from build123d import *

# Parameters (mm, degrees)
F2_R     = 8
F3_SIZE2 = 13
F3_SIZE  = 4


with BuildPart() as f1:
    # F0 (on Top) → F1 (revolve)
    with BuildSketch(Plane.XY):
        with BuildLine():
            Line((-14.3607687205, 22), (-14.3607687205, -20))
            Line((-14.3607687205, -20), (32.0355594158, -20))
            Line((32.0355594158, -20), (32.0355594158, 9.6684019268))
            Line((32.0355594158, 9.6684019268), (52.5324852616, 9.6684019268))
            Line((52.5324852616, 9.6684019268), (52.5324852616, 46.7559769824))
            ThreePointArc((52.5324852616, 46.7559769824), (51.0680191675, 50.2915108883), (47.5324852616, 51.7559769824))
            Line((47.5324852616, 51.7559769824), (16.6392312795, 51.7559769824))
            Line((16.6392312795, 51.7559769824), (16.6392312795, 22))
            Line((16.6392312795, 22), (-14.3607687205, 22))
        make_face()
    revolve(axis=Axis((-14.3607687205, 1, 0), (0, -1, 0)))

    # F2
    f2_edges = [f1.edges().sort_by_distance(p)[0] for p in [
        (-45.360769, 51.755977, 0),
    ]]
    fillet(f2_edges, radius=F2_R)

    # F3
    f3_edges = [f1.edges().sort_by_distance(p)[0] for p in [
        (-60.757097, -20, 0),
    ]]
    chamfer(f3_edges, length=F3_SIZE, length2=F3_SIZE2)


solid = f1.part
For this review, take the finished solid that the model builds, in its own axes (mm). A direction names the side the tool comes from. Round coordinates to 2 decimals unless told otherwise and drop trailing zeros. Order: outer loops, then holes, each group sorted by start corner. A loop starts at its lowest first (then second) coordinate and runs counter-clockwise, first axis right, second up. Notation, with made-up numbers: M -28,40 L -7,40 A26 ccw -7,57 Z; hole C 7.25,56 d5. An arc over 180 degrees is marked long. Use a Markdown table: item, result. Add a question column.
Item 1: Add section A-A, the plane z = 0. Give the boundary of the cut face in (x, y), then the cut area to 3 significant figures.
Item 2: Tool access review of faces 1 (the flat face through (-15, 51.756, -40)), 2 (the cylindrical face through (-60.712, -2.986, 2.04)): name each direction out of +Z, -Z, +X, -X, +Y, -Y from which nothing blocks a thin tool from reaching the whole face with its end or side.
Item 3: Add section D-D, the plane y = 4. Give the boundary of the cut face in (x, z), then the cut area to 3 significant figures.
Item 4: To check wall thickness, follow line 1 along Y through (x, z) = (39.5, -27.5); line 2 along Z through (x, y) = (-16, 38.5); line 3 along Z through (x, y) = (-26.5, 49.5). State the ranges of each line that lie inside material, in increasing order.
Item 5: Add section C-C, the plane y = 14. Give the boundary of the cut face in (x, z), then the cut area to 3 significant figures.
Item 6: Insertion check: pin 1 (2 mm diameter, centred on x = -56, y = 40, fed in from +Z); pin 2 (8 mm diameter, centred on y = 24, z = -16, fed in from +X); pin 3 (10 mm diameter, centred on x = -13.5, y = 42, fed in from -Z). Each pin has a flat end and moves straight along its axis. Give the tip position at first contact, or say it passes through.
Item 7: Add section B-B, the plane y = 40. Give the boundary of the cut face in (x, z).
Item 8: Mouldability with a two-part tool opening along Z and no side actions: class faces 3 (the flat face through (-15, 22, 0)), 4 (the conical face through (-21.737, -19.806, -33.218)), 5 (the cylindrical face through (2.3, 32.73, 26.14)), 6 (the flat face through (1, 9.668, -44)) as released by +Z, released by -Z, zero draft, split by the parting line, or undercut.
Geometry results:
| question | item | result |
|---|---|---|
| 1 | outline | M -81.25,9.67 L -60.76,9.67 L -60.76,-16 L -47.76,-20 L 19.04,-20 L 32.04,-16 L 32.04,9.67 L 52.53,9.67 L 52.53,46.76 A5 ccw 47.53,51.76 L 24.64,51.76 A8 ccw 16.64,43.76 L 16.64,22 L -45.36,22 L -45.36,43.76 A8 ccw -53.36,51.76 L -76.25,51.76 A5 ccw -81.25,46.76 Z |
| 1 | area | 6,450 mm² |
| 2 | face 1 | +Z, -Z, +X, -X, +Y |
| 2 | face 2 | -Y |
| 3 | outline | C -14.36,0 d92.79 |
| 3 | area | 6,760 mm² |
| 4 | line 1 | y = 9.67 to 51.76 |
| 4 | line 2 | z = -66.87 to -30.96, 30.96 to 66.87 |
| 4 | line 3 | z = -64.95 to -31.15, 31.15 to 64.95 |
| 5 | outline | C -14.36,0 d133.79 |
| 5 | area | 14,100 mm² |
| 6 | pin 1 | stops at z = 53.13 |
| 6 | pin 2 | stops at x = 51.45 |
| 6 | pin 3 | stops at z = -66.89 |
| 7 | outline | C -14.36,0 d133.79; hole C -14.36,0 d62 |
| 8 | face 3 | undercut |
| 8 | face 4 | split by the parting line |
| 8 | face 5 | undercut |
| 8 | face 6 | zero draft |
